```python
from build123d import *

# Parameters (mm, degrees)
BOSS_EXTRU_1_DEPTH      = 30
ESQUISSE2_R             = 1.75
ENL_V_MAT_EXTRU_1_DEPTH = 37.551333765
ESQUISSE3_R             = 3
ENL_V_MAT_EXTRU_2_DEPTH = 2.5
ESQUISSE4_W             = 30
ESQUISSE4_H             = 10
ESQUISSE4_R             = 2
BOSS_EXTRU_2_DEPTH      = 4
ESQUISSE5_W             = 9.5
ESQUISSE5_H             = 12.5
ESQUISSE5_H_2           = 10
BOSS_EXTRU_3_DEPTH      = 10
ESQUISSE6_R             = 3
ENL_V_MAT_EXTRU_3_DEPTH = 8


with BuildPart() as part:
    # Esquisse1 → Boss.-Extru.1 (new body)
    with BuildSketch(Plane.XY):
        Polygon((9.5, 20), (9.5, 17.5), (3.5, 17.5), (3.5, 2.5), (9.5, 2.5), (9.5, 0), (0, 0), (0, 20), align=None)
    extrude(amount=BOSS_EXTRU_1_DEPTH)

    # Esquisse2 → Enlèv. mat.-Extru.1 (cut, through all)
    with BuildSketch(Plane(origin=(3.5, 0, 0), x_dir=(0, 0, -1), z_dir=(1, 0, 0))):
        with Locations((-22, 10)):
            Circle(ESQUISSE2_R)
        with Locations((-8, 10)):
            Circle(ESQUISSE2_R)
    extrude(amount=-ENL_V_MAT_EXTRU_1_DEPTH, mode=Mode.SUBTRACT)

    # Esquisse3 → Enlèv. mat.-Extru.2 (cut)
    with BuildSketch(Plane.ZY):
        with Locations((8, 10)):
            Circle(ESQUISSE3_R)
        with Locations((22, 10)):
            Circle(ESQUISSE3_R)
    extrude(amount=-ENL_V_MAT_EXTRU_2_DEPTH, mode=Mode.SUBTRACT)

    # Esquisse4 → Boss.-Extru.2 (add)
    # profile 1 of 2: a face of its own
    with BuildSketch(Plane.ZY):
        with Locations((15, -5)):
            Rectangle(ESQUISSE4_W, ESQUISSE4_H)
        with Locations((15, -5)):
            Circle(ESQUISSE4_R, mode=Mode.SUBTRACT)
        with Locations((5, -5)):
            Circle(ESQUISSE4_R, mode=Mode.SUBTRACT)
        with Locations((25, -5)):
            Circle(ESQUISSE4_R, mode=Mode.SUBTRACT)
    # profile 2 of 2: a face of its own
    with BuildSketch(Plane.ZY):
        with Locations((15, 25)):
            Rectangle(ESQUISSE4_W, ESQUISSE4_H)
        with Locations((15, 25)):
            Circle(ESQUISSE4_R, mode=Mode.SUBTRACT)
        with Locations((5, 25)):
            Circle(ESQUISSE4_R, mode=Mode.SUBTRACT)
        with Locations((25, 25)):
            Circle(ESQUISSE4_R, mode=Mode.SUBTRACT)
    extrude(amount=-BOSS_EXTRU_2_DEPTH)

    # Esquisse5 → Boss.-Extru.3 (add)
    with BuildSketch(Plane(origin=(0, 0, 0), x_dir=(-1, 0, 0), z_dir=(0, 0, -1))):
        with Locations((-4.75, 23.75)):
            Rectangle(ESQUISSE5_W, ESQUISSE5_H)
        with Locations((-4.75, -5)):
            Rectangle(ESQUISSE5_W, ESQUISSE5_H_2)
    extrude(amount=-BOSS_EXTRU_3_DEPTH)

    # Esquisse6 → Enlèv. mat.-Extru.3 (cut)
    with BuildSketch(Plane(origin=(0, 0, 0), x_dir=(-1, 0, 0), z_dir=(0, 0, -1))):
        with Locations((-5, 25)):
            Circle(ESQUISSE6_R)
        with Locations((-5, -5)):
            Circle(ESQUISSE6_R)
    extrude(amount=-ENL_V_MAT_EXTRU_3_DEPTH, mode=Mode.SUBTRACT)


solid = part.part
```
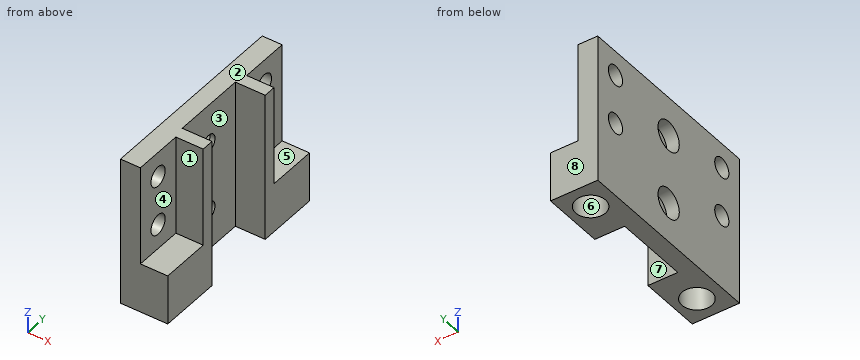
For this review, take the finished solid that the model builds, in its own axes (mm). Face numbers are marked on the shaded views. A direction names the side the tool comes from. Coordinates: 2 decimals unless noted, no trailing zeros. Write each loop counter-clockwise with the first axis right and the second up, starting at its lowest first coordinate (ties: lowest second). Pieces come first, ordered by that corner, then holes. Notation, with made-up numbers: (-22.75, 12) - (30.25, 12) arc R9 ccw to (30.25, 23) - close; hole circle Ø5 at (84, 14). An arc over 180 degrees is marked (long way). Put each result on its own line as item: value.
1. Wall thickness on probe 1 along Y at (x, z) = (5, 5.5); probe 2 along Y at (x, z) = (1.85, 15); probe 3 along Y at (x, z) = (5.25, 27.25): over which ranges is each line inside the solid? List them lowest first.
Values found:
probe 1: -10 to -8, -2 to 2.5, 17.5 to 22, 28 to 30
probe 2: -10 to -7, -3 to 23, 27 to 30
probe 3: 0 to 2.5, 17.5 to 20
2. Add section D-D, the plane y = 10. Give the boundary of the cut face in (x, z).
Values found:
outline: (0, 0) - (3.5, 0) - (3.5, 6.25) - (2.5, 6.25) - (2.5, 5) - (0, 5) - close; (0, 11) - (2.5, 11) - (2.5, 9.75) - (3.5, 9.75) - (3.5, 20.25) - (2.5, 20.25) - (2.5, 19) - (0, 19) - close; (0, 25) - (2.5, 25) - (2.5, 23.75) - (3.5, 23.75) - (3.5, 30) - (0, 30) - close
3. Mouldability with a two-part tool opening along Y and no side actions: class the marked faces 1, 2 and 3 as released by +Y, released by -Y, zero draft, split by the parting line, or undercut.
Values found:
face 1: released by -Y
face 2: zero draft
face 3: undercut
4. Add section A-A, the plane x = 5. Give the boundary of the cut face in (y, z).
Values found:
outline: (-10, 0) - (-8, 0) - (-8, 8) - (-2, 8) - (-2, 0) - (2.5, 0) - (2.5, 30) - (0, 30) - (0, 10) - (-10, 10) - close; (17.5, 0) - (22, 0) - (22, 8) - (28, 8) - (28, 0) - (30, 0) - (30, 10) - (20, 10) - (20, 30) - (17.5, 30) - close
5. Add section C-C, the plane x = 1.25. Give the boundary of the cut face in (y, z), then the cut area to 3 significant figures.
Values found:
outline: (-10, 0) - (30, 0) - (30, 30) - (-10, 30) - close; hole circle Ø4 at (-5, 15); hole circle Ø4 at (-5, 25); hole circle Ø6 at (10, 8); hole circle Ø6 at (10, 22); hole circle Ø4 at (25, 15); hole circle Ø4 at (25, 25)
area: 1,090 mm²
6. Add section B-B, the plane z = 15. Give the boundary of the cut face in (x, y).
Values found:
outline: (0, -10) - (4, -10) - (4, -7) - (0, -7) - close; (0, -3) - (4, -3) - (4, 0) - (9.5, 0) - (9.5, 2.5) - (3.5, 2.5) - (3.5, 17.5) - (9.5, 17.5) - (9.5, 20) - (4, 20) - (4, 23) - (0, 23) - close; (0, 27) - (4, 27) - (4, 30) - (0, 30) - close
7. Machinability: for the marked faces 4, 5, 6, 7 and 8, which of the approach directions +Z, -Z, +X, -X, +Y, -Y give a long, thin tool a straight path to every point of the face, cutting with its end or side? Answer none if there is none.
Values found:
face 4: +Z, +X, -Y
face 5: +Z, +X, +Y
face 6: -Z
face 7: +Z, -Z, +X
face 8: +Z, -Z, +X, -X, +Y
8. For pin 1 (3 mm diameter, centred on x = 6.5, y = 25.5, fed in from +Z); pin 2 (5 mm diameter, centred on x = 6.5, y = 14, fed in from -Z); pin 3 (3 mm diameter, centred on y = 10.5, z = 21.5, fed in from -X); pin 4 (3 mm diameter, centred on y = -5.5, z = 19, fed in from +X), all flat-tipped, find the tip position at first contact; note any pin that passes through.
Values found:
pin 1: z = 10
pin 2: through
pin 3: x = 2.5
pin 4: x = 4
